Autodesk Inventor part; units mm, degrees
ref_plane "Start plane" through (0, 0, -17.5) normal (0, 0, 1) x (1, 0, 0)
ref_plane "End plane" through (0, 0, 497.5) normal (0, 0, 1) x (1, 0, 0)
ref_plane "Work Plane4" through (107.5, 0, -17.5) normal (0, 0, -1) x (-1, 0, 0)
ref_plane "Start plane" through (0, 0, -17.5) normal (0, 0, 1) x (1, 0, 0)
ref_plane "End plane" through (0, 0, 497.5) normal (0, 0, 1) x (1, 0, 0)
sketch "Sketch" plane through (0, 0, 0) normal (0, 0, 1) x (1, 0, 0)
  line L0 (-17.5, -12.5) -> (-17.5, 12.5)
  line L1 (-12.5, 17.5) -> (12.5, 17.5)
  line L2 (17.5, 12.5) -> (17.5, -12.5)
  line L3 (12.5, -17.5) -> (-12.5, -17.5)
  arc A0 (-17.5, -12.5) -> (-12.5, -17.5) centre (-12.5, -12.5) ccw
  arc A1 (-12.5, 17.5) -> (-17.5, 12.5) centre (-12.5, 12.5) ccw
  arc A2 (17.5, 12.5) -> (12.5, 17.5) centre (12.5, 12.5) ccw
  arc A3 (12.5, -17.5) -> (17.5, -12.5) centre (12.5, -12.5) ccw
  arc A4 (-12.5, 15) -> (-15, 12.5) centre (-12.5, 12.5) ccw
  line L4 (-12.5, 15) -> (12.5, 15)
  arc A5 (15, 12.5) -> (12.5, 15) centre (12.5, 12.5) ccw
  line L5 (15, 12.5) -> (15, -12.5)
  arc A6 (12.5, -15) -> (15, -12.5) centre (12.5, -12.5) ccw
  line L6 (12.5, -15) -> (-12.5, -15)
  arc A7 (-15, -12.5) -> (-12.5, -15) centre (-12.5, -12.5) ccw
  line L7 (-15, -12.5) -> (-15, 12.5)
  line L8 (0, 25.9497) -> (0, -25.9497) construction
  line L9 (-25.9497, 0) -> (25.9497, 0) construction
  dimension "d7" = 5
  dimension "d10" = 35
  dimension "d11" = 35
  dimension "d12" = 2.5
  dimension "d15" = 17.5
  dimension "d16" = 17.5
extrude "Body" add sketch "Sketch" along normal up to surface (515 mm away) from surface at -17.5
sketch "Sketch3" plane through (0, 0, 0) normal (0, 0, 1) x (1, 0, 0)
  line L0 (0, 0) -> (10, 0)
ref_plane "Work Plane3" through (0, 0, 0) normal (0, -1, 0) x (1, 0, 0)
sketch "Sketch4" plane through (0, 0, 0) normal (0, -1, 0) x (1, 0, 0)
  line L0 (-2, -17.5) -> (12, -17.5)
  line L1 (-2, 497.5) -> (12, 497.5)
  dimension "d18" = 515
ref_plane "Work Plane4" through (107.5, 0, -17.5) normal (0, 0, -1) x (-1, 0, 0)
split "Split1" plane through (107.5, 0, -17.5) removes the side toward (0, 0, -1)
ref_plane "Work Plane5" through (0, -17.5, 497.5) normal (0, 0.7071, 0.7071) x (1, 0, 0)
split "Split2" plane through (0, -17.5, 497.5) removes the side toward (0, 0.7071, 0.7071)
ref_plane "Work Plane7" through (0, 780, 380) normal (0, -1, 0) x (1, 0, 0)
ref_plane "Work Plane8" through (0, 0, 380) normal (0, -1, 0) x (1, 0, 0)
ref_plane "Work Plane9" through (0, 390, 380) normal (0, -1, 0) x (1, 0, 0)
ref_plane "Work Plane10" through (0, 0, 100) normal (0, 1, 0) x (-1, 0, 0)
ref_plane "Work Plane11" through (0, 780, 100) normal (0, 1, 0) x (-1, 0, 0)
ref_plane "Work Plane12" through (0, 390, 100) normal (0, 1, 0) x (-1, 0, 0)
ref_plane "Work Plane13" through (0, -17.5, -17.5) normal (0, 0.7071, -0.7071) x (1, 0, 0)
split "Split4" plane through (0, -17.5, -17.5) removes the side toward (0, 0.7071, -0.7071)
sketch "Sketch5" plane through (0, 390, 380) normal (0, -1, 0) x (1, 0, 0)
  arc A0 (-17.5, -12.5) -> (-12.5, -17.5) centre (-12.5, -12.5) ccw
  line L0 (-17.5, -12.5) -> (-17.5, 12.5)
  arc A1 (-12.5, 17.5) -> (-17.5, 12.5) centre (-12.5, 12.5) ccw
  line L1 (-12.5, 17.5) -> (12.5, 17.5)
  arc A2 (17.5, 12.5) -> (12.5, 17.5) centre (12.5, 12.5) ccw
  line L2 (17.5, 12.5) -> (17.5, -12.5)
  arc A3 (12.5, -17.5) -> (17.5, -12.5) centre (12.5, -12.5) ccw
  line L3 (12.5, -17.5) -> (-12.5, -17.5)
  arc A4 (-12.5, 15) -> (-15, 12.5) centre (-12.5, 12.5) ccw
  line L4 (-12.5, 15) -> (12.5, 15)
  arc A5 (15, 12.5) -> (12.5, 15) centre (12.5, 12.5) ccw
  line L5 (15, 12.5) -> (15, -12.5)
  arc A6 (12.5, -15) -> (15, -12.5) centre (12.5, -12.5) ccw
  line L6 (12.5, -15) -> (-12.5, -15)
  arc A7 (-15, -12.5) -> (-12.5, -15) centre (-12.5, -12.5) ccw
  line L7 (-15, -12.5) -> (-15, 12.5)
extrude "Extrusion2" cut sketch "Sketch5" along normal up to surface (780 mm away) from surface at -390 contours L0 A1 L1 A2 L2 A3 L3 A0 | L4 A5 L5 A6 L6 A7 L7 A4
sketch "Sketch6" plane through (0, 390, 100) normal (0, 1, 0) x (-1, 0, 0)
  arc A0 (-17.5, -12.5) -> (-12.5, -17.5) centre (-12.5, -12.5) ccw
  line L0 (-17.5, -12.5) -> (-17.5, 12.5)
  arc A1 (-12.5, 17.5) -> (-17.5, 12.5) centre (-12.5, 12.5) ccw
  line L1 (-12.5, 17.5) -> (12.5, 17.5)
  arc A2 (17.5, 12.5) -> (12.5, 17.5) centre (12.5, 12.5) ccw
  line L2 (17.5, 12.5) -> (17.5, -12.5)
  arc A3 (12.5, -17.5) -> (17.5, -12.5) centre (12.5, -12.5) ccw
  line L3 (12.5, -17.5) -> (-12.5, -17.5)
  arc A4 (-12.5, 15) -> (-15, 12.5) centre (-12.5, 12.5) ccw
  line L4 (-12.5, 15) -> (12.5, 15)
  arc A5 (15, 12.5) -> (12.5, 15) centre (12.5, 12.5) ccw
  line L5 (15, 12.5) -> (15, -12.5)
  arc A6 (12.5, -15) -> (15, -12.5) centre (12.5, -12.5) ccw
  line L6 (12.5, -15) -> (-12.5, -15)
  arc A7 (-15, -12.5) -> (-12.5, -15) centre (-12.5, -12.5) ccw
  line L7 (-15, -12.5) -> (-15, 12.5)
extrude "Extrusion3" cut sketch "Sketch6" along normal up to surface (780 mm away) from surface at -390 contours L0 A1 L1 A2 L2 A3 L3 A0 | L4 A5 L5 A6 L6 A7 L7 A4
equation "\"d7\" = G_IR"
equation "\"d10\" = G_H"
equation "\"d11\" = G_W"
equation "\"d12\" = G_T"
equation "\"d15\" = 0.5 * d10"
equation "\"d16\" = 0.5 * d11"
equation "\"d3\" = G_L"
equation "\"G_W\" = 35"
equation "\"G_H\" = 35"
equation "\"G_T\" = 2.5"
equation "\"G_IR\" = 5"
equation "\"G_L\" = d18"
equation "\"G_OFFSET_START\" = 17.5"
equation "\"G_OFFSET_END\" = 17.5"
equation "\"d13\" = -G_OFFSET_START"
equation "\"d14\" = G_OFFSET_END + B_L"
properties part number "AS 1163 - C350L0 35x35x2.5 SHS - 515" material "Steel, Mild"
The model under review builds one solid part; all positions refer to its coordinate system, in mm. A direction names the side the tool comes from. Round coordinates to 2 decimals unless told otherwise and drop trailing zeros. Loops run counter-clockwise (first coordinate to the right, second up) from the corner with the lowest first, then second, coordinate; pieces in that order, holes last. Notation, with made-up numbers: (14.5, -13) - (19.5, -13) arc R10 cw to (19.5, 4) - close; hole circle Ø5 at (14.5, 12). An arc over 180 degrees is marked (long way). Write each question's results on one line, items separated by ' | '. Start each with the question number.
Q1. Wall thickness on line 1 along X through (y, z) = (9, 227); line 2 along Z through (x, y) = (15.5, 4.5): over which ranges is each line inside the solid? List them lowest first. Write a range as [from, to].
Q2. Take a section at B-B on x = 3. Give the boundary of the cut face in (y, z).
Q3. Take a section at A-A on y = -5. Give the boundary of the cut face in (x, z).
Q4. Take a section at C-C on z = 70. Give the boundary of the cut face in (x, y).
Q5. Tool access review of faces 4 (the flat face through (0, -15, 236)), 5 (the flat face through (15.3, 0.2, 0.2)): name each direction out of +Z, -Z, +X, -X, +Y, -Y from which nothing blocks a thin tool from reaching the whole face with its end or side.
Q6. Draft analysis for pull direction Y (two halves, no side actions). For faces 1 (the flat face through (-17.5, 0, 236)), 2 (the flat face through (0, 17.5, 430)), 3 (the flat face through (0, 15, 238)), state which applies: pulls with the +Y half, pulls with the -Y half, needs draft (parallel to the pull), parting line crosses it, or undercut.
Q7. Insertion check: P1, Ø1.2, axis at x = -16, z = 108, coming from the +Y side; P2, Ø1.2, axis at x = 6, y = 16, coming from the -Z side; P3, Ø1, axis at x = -13, y = -5, coming from the +Z side; P4, Ø3, axis at x = 3.5, y = 16, coming from the +Z side. Each pin has a flat end and moves straight along its axis. Give the tip position at first contact, or say it passes through.
Data:
1) line 1: x = [-17.5, -15], [15, 17.5] | line 2: z = [4.5, 83.5], [116.5, 363.5], [396.5, 475.5]
2) outline: (-17.5, -17.5) - (-15, -15) - (-15, 495) - (-17.5, 497.5) - close; (15, 15) - (17.5, 17.5) - (17.5, 82.5) - (15, 82.5) - close; (15, 117.5) - (17.5, 117.5) - (17.5, 362.5) - (15, 362.5) - close; (15, 397.5) - (17.5, 397.5) - (17.5, 462.5) - (15, 465) - close
3) outline: (-17.5, -5) - (-15, -5) - (-15, 485) - (-17.5, 485) - close; (15, -5) - (17.5, -5) - (17.5, 485) - (15, 485) - close
4) outline: (-17.5, -12.5) arc R5 ccw to (-12.5, -17.5) - (12.5, -17.5) arc R5 ccw to (17.5, -12.5) - (17.5, 12.5) arc R5 ccw to (12.5, 17.5) - (-12.5, 17.5) arc R5 ccw to (-17.5, 12.5) - close; hole (-15, -12.5) arc R2.5 ccw to (-12.5, -15) - (12.5, -15) arc R2.5 ccw to (15, -12.5) - (15, 12.5) arc R2.5 ccw to (12.5, 15) - (-12.5, 15) arc R2.5 ccw to (-15, 12.5) - close
5) face 4: +Z, -Z | face 5: -Z, +X, -X, +Y
6) face 1: needs draft | face 2: pulls with the +Y half | face 3: undercut
7) P1: stops at y = 0 | P2: stops at z = 15.4 | P3: passes through | P4: stops at z = 465
